For this review, take the finished solid that the model builds, in its own axes (mm). Coordinates: 2 decimals unless noted, no trailing zeros. Loops run counter-clockwise (first coordinate to the right, second up) from the corner with the lowest first, then second, coordinate; pieces in that order, holes last. Notation, with made-up numbers: (89.5, -13) - (115.5, -13) arc R20 cw to (115.5, 5) - close; hole circle Ø1 at (-9.75, -28). An arc over 180 degrees is marked (long way). Use one line per item in the form item = value. Start each with the question number.
1. Add section A-A on y = 1.15. Give the boundary of the cut face in (x, z).
2. To check wall thickness, follow probe 1 along Z at (x, y) = (-2, 0); probe 2 along X at (y, z) = (-0.5, 90.5); probe 3 along X at (y, z) = (1.25, 226). State the ranges of each line that lie inside material, in increasing order.
3. For pin 1 Ø2 at (x, y) = (145.5, 1) entering from -Z; pin 2 Ø2 at (y, z) = (-1.5, 154) entering from -X; pin 3 Ø1.8 at (y, z) = (1, 5) entering from +X, all flat-tipped, find the tip position at first contact; note any pin that passes through.
```python
from build123d import *

# Parameters (mm, degrees)
SKETCH1_W           = 10
SKETCH1_H           = 6
SKETCH5_R           = 2.5
CUT_EXTRUDE1_DEPTH  = 17.997170664
SKETCH6_R           = 2.5
BOSS_EXTRUDE1_DEPTH = 330


with BuildPart() as part:
    # Sweep2: sweep along a path in Sketch4
    with BuildLine(Plane(origin=(0, 0, 0), x_dir=(1, 0, 0), z_dir=(0, 1, 0))) as sweep2_path:
        Line((0, 0), (0, -5))
        Line((0, -5), (2.5, -9.330127019))
    # Sketch1 → Sweep2 (sweep)
    with BuildSketch(Plane.XY):
        Rectangle(SKETCH1_W, SKETCH1_H)
    sweep(path=sweep2_path.line, transition=Transition.RIGHT)

    # Sketch5 → Cut-Extrude1 (cut, through all)
    with BuildSketch(Plane.ZY.offset(5)):
        with Locations(Location((3.245776798, 0, 0), (0, 0, 270))):
            Circle(SKETCH5_R)
    extrude(amount=-CUT_EXTRUDE1_DEPTH, mode=Mode.SUBTRACT)

    # SurfaceCut1
    split(bisect_by=Plane(origin=(5, 0, 0), x_dir=(0, 0, -1), z_dir=(1, 0, 0)), keep=Keep.BOTTOM)

    # Sketch6 → Boss-Extrude1 (add)
    with BuildSketch(Plane(origin=(4.665063509, 0, 8.080127019), x_dir=(0.8660254037844379, 0, -0.5000000000000013), z_dir=(0.5000000000000012, 0, 0.8660254037844378))):
        with Locations((-4.837322129, 0)):
            Circle(SKETCH6_R)
    extrude(amount=BOSS_EXTRUDE1_DEPTH)


solid = part.part
```
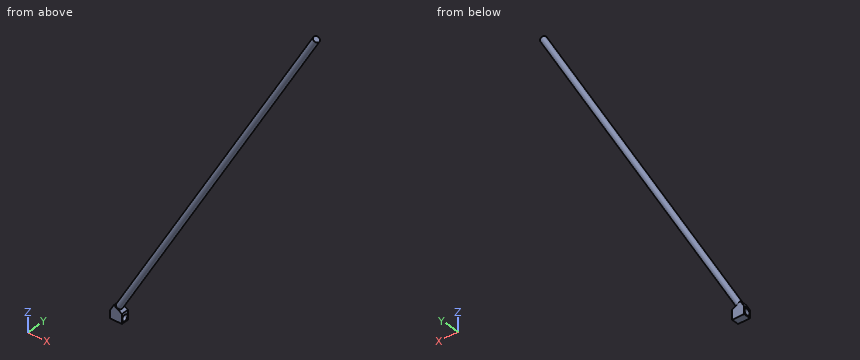
Conclusion:
q1.outline = (-5, 0) - (5, 0) - (5, 1.03) - (-5, 1.03) - close; (-5, 5.47) - (5, 5.47) - (5, 7.89) - (2.4, 9.39) - (167.4, 295.18) - (163.55, 297.4) - (-1.45, 11.61) - (-1.83, 11.83) - (-5, 6.34) - close
q2.probe_1 = 0 to 0.75, 5.75 to 11.54
q2.probe_2 = 43.84 to 49.49
q2.probe_3 = 122.4 to 127.4
q3.pin_1 = 255.24
q3.pin_2 = 80.17
q3.pin_3 = 5
